Geometry check sheet. Reference: the model listing, model coordinates, mm. A direction names the side the tool comes from. Coordinates: 2 decimals unless noted, no trailing zeros. Write each loop counter-clockwise with the first axis right and the second up, starting at its lowest first coordinate (ties: lowest second). Pieces come first, ordered by that corner, then holes. Notation, with made-up numbers: M -13,-40 L 20,-40 A20 ccw 20,-33 Z; hole C 36,18 d9. An arc over 180 degrees is marked long. Put each result on its own line as item: value. Start each with the question number.
1) Mould release check, pull along X, two halves, no side actions. Record for faces 4 (the cylindrical face through (39.86, 32.907, 10.363)), 5 (the cylindrical face through (32.53, -29.11, 26.7)), 6 (the flat face through (50, 23, -26)): released by +X, released by -X, zero draft, split by the parting line, or undercut.
2) Gauge pin test, flat ends, axial feed: pin 1 (1 mm diameter, centred on x = 36, y = -24.5, fed in from -Z); pin 2 (5 mm diameter, centred on x = 40.5, z = 9, fed in from +Y); pin 3 (12 mm diameter, centred on y = -16.5, z = -4.5, fed in from -X); pin 4 (4 mm diameter, centred on x = 15.5, z = -35.5, fed in from -Y). Record the tip position at first contact, or that the pin passes through.
3) Cross-section at C-C on x = 37. Record the cut outline in (y, z).
4) Cross-section at A-A on y = 0. Record the cut outline in (x, z).
5) Cross-section at D-D on x = 19. Record the cut outline in (y, z).
6) Set-up check for faces 1 (the flat face through (45, 17, -36)), 2 (the flat face through (30, 0, 0)), 3 (the flat face through (0, 1, 1)): record each of +Z, -Z, +X, -X, +Y, -Y from which the full face is reachable in a straight line by a thin tool's end or side.
7) Scan lines: line 1 along X through (y, z) = (-36.5, -23.5); line 2 along Z through (x, y) = (37, 0); line 3 along X through (y, z) = (6, 11.5). Record each from-to range of solid material in increasing order.
from build123d import *


with BuildPart() as part:
    # Sketch1 → Revolve1 (revolve)
    with BuildSketch(Plane.XY):
        Polygon((0, 0), (0, 44.5), (30, 44.5), (30, 39.5), (35, 39.5), (35, 44.5), (40, 44.5), (40, 39.5), (45, 39.5), (45, 44.5), (50, 44.5), (50, 34.5), (30, 34.5), (30, 0), align=None)
    revolve(axis=Axis((0, 0, 0), (1, 0, 0)))


solid = part.part
Answer key:
1. face 4: zero draft
1. face 5: undercut
1. face 6: released by +X
2. pin 1: stops at z = -37.47
2. pin 2: stops at y = 44.02
2. pin 3: stops at x = 0
2. pin 4: stops at y = -29.29
3. outline: C 0,0 d89; hole C 0,0 d69
4. outline: M 0,-44.5 L 30,-44.5 L 30,-39.5 L 35,-39.5 L 35,-44.5 L 40,-44.5 L 40,-39.5 L 45,-39.5 L 45,-44.5 L 50,-44.5 L 50,-34.5 L 30,-34.5 L 30,34.5 L 50,34.5 L 50,44.5 L 45,44.5 L 45,39.5 L 40,39.5 L 40,44.5 L 35,44.5 L 35,39.5 L 30,39.5 L 30,44.5 L 0,44.5 Z
5. outline: C 0,0 d89
6. face 1: none
6. face 2: +X
6. face 3: +Z, -Z, -X, +Y, -Y
7. line 1: x = 0 to 30, 35 to 40, 45 to 50
7. line 2: z = -44.5 to -34.5, 34.5 to 44.5
7. line 3: x = 0 to 30
